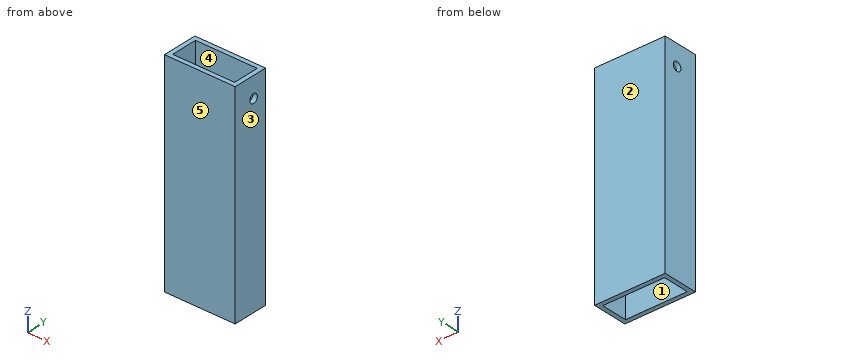
from build123d import *

# Parameters (mm, degrees)
SKETCH1_W           = 50.8
SKETCH1_H           = 25.4
SKETCH1_W_2         = 44.45
SKETCH1_H_2         = 19.05
BOSS_EXTRUDE1_DEPTH = 152.4
SKETCH2_R           = 3.175
CUT_EXTRUDE1_DEPTH  = 162.144934764


with BuildPart() as part:
    # Sketch1 → Boss-Extrude1 (new body)
    with BuildSketch(Plane.XY):
        Rectangle(SKETCH1_W, SKETCH1_H)
        Rectangle(SKETCH1_W_2, SKETCH1_H_2, mode=Mode.SUBTRACT)
    extrude(amount=BOSS_EXTRUDE1_DEPTH)

    # Sketch2 → Cut-Extrude1 (cut, through all)
    with BuildSketch(Plane(origin=(25.4, 0, 0), x_dir=(0, 0, -1), z_dir=(1, 0, 0))):
        with Locations((-137.513740162, 2.738654121)):
            Circle(SKETCH2_R)
    extrude(amount=-CUT_EXTRUDE1_DEPTH, mode=Mode.SUBTRACT)


solid = part.part
The model under review builds one solid part; all positions refer to its coordinate system, in mm. Face numbers are marked on the shaded views. A direction names the side the tool comes from. Coordinates: 2 decimals unless noted, no trailing zeros. Order: outer loops, then holes, each group sorted by start corner. A loop starts at its lowest first (then second) coordinate and runs counter-clockwise, first axis right, second up. Notation, with made-up numbers: (7.25, -13) -> (31.25, -13) arc R34 cw to (31.25, 25) -> close; hole circle Ø10 at (-22.75, 6.25). An arc over 180 degrees is marked (long way). Answer in a Markdown table with one row per item.
(1) Machinability: for the marked faces 1 and 2, which of the approach directions +Z, -Z, +X, -X, +Y, -Y give a long, thin tool a straight path to every point of the face, cutting with its end or side? Answer none if there is none.
Answers:
| item | result |
|---|---|
| face 1 | +Z, -Z |
| face 2 | +Z, -Z, +X, -X, +Y |
(2) Consider section A-A (x = 11). Write out the cut boundary in (y, z) (3 decimals).
Answers:
| item | result |
|---|---|
| outline | (-12.7, 0) -> (-9.525, 0) -> (-9.525, 152.4) -> (-12.7, 152.4) -> close; (9.525, 0) -> (12.7, 0) -> (12.7, 152.4) -> (9.525, 152.4) -> close |
(3) Insertion check: pin 1 (5 mm diameter, centred on y = 2.74, z = 137.51, fed in from +X). The pin has a flat end and moves straight along its axis. Give the tip position at first contact, or say it passes through.
Answers:
| item | result |
|---|---|
| pin 1 | through |
(4) Wall thickness on line 1 along X through (y, z) = (-1.5, 102.5) (3 decimals); line 2 along Y through (x, z) = (-22, 62) (3 decimals): over which ranges is each line inside the solid? List them lowest first.
Answers:
| item | result |
|---|---|
| line 1 | -25.4 to -22.225, 22.225 to 25.4 |
| line 2 | -12.7 to -9.525, 9.525 to 12.7 |
(5) Consider section B-B (y = 8). Write out the cut boundary in (x, z) (3 decimals), plus the area to 3 significant figures.
Answers:
| item | result |
|---|---|
| outline | (-25.4, 0) -> (-22.225, 0) -> (-22.225, 152.4) -> (-25.4, 152.4) -> close; (22.225, 0) -> (25.4, 0) -> (25.4, 152.4) -> (22.225, 152.4) -> close |
| area | 968 mm² |
(6) Consider section C-C (z = 129.5). Write out the cut boundary in (x, y) (3 decimals).
Answers:
| item | result |
|---|---|
| outline | (-25.4, -12.7) -> (25.4, -12.7) -> (25.4, 12.7) -> (-25.4, 12.7) -> close; hole (-22.225, -9.525) -> (22.225, -9.525) -> (22.225, 9.525) -> (-22.225, 9.525) -> close |
(7) The part is to be moulded in two halves that separate along X. For the marked faces 3, 4 and 5, say which applies: +X half, -X half, draft (parallel to the pull), parting line (faces both ways), or undercut.
Answers:
| item | result |
|---|---|
| face 3 | +X half |
| face 4 | undercut |
| face 5 | draft |
